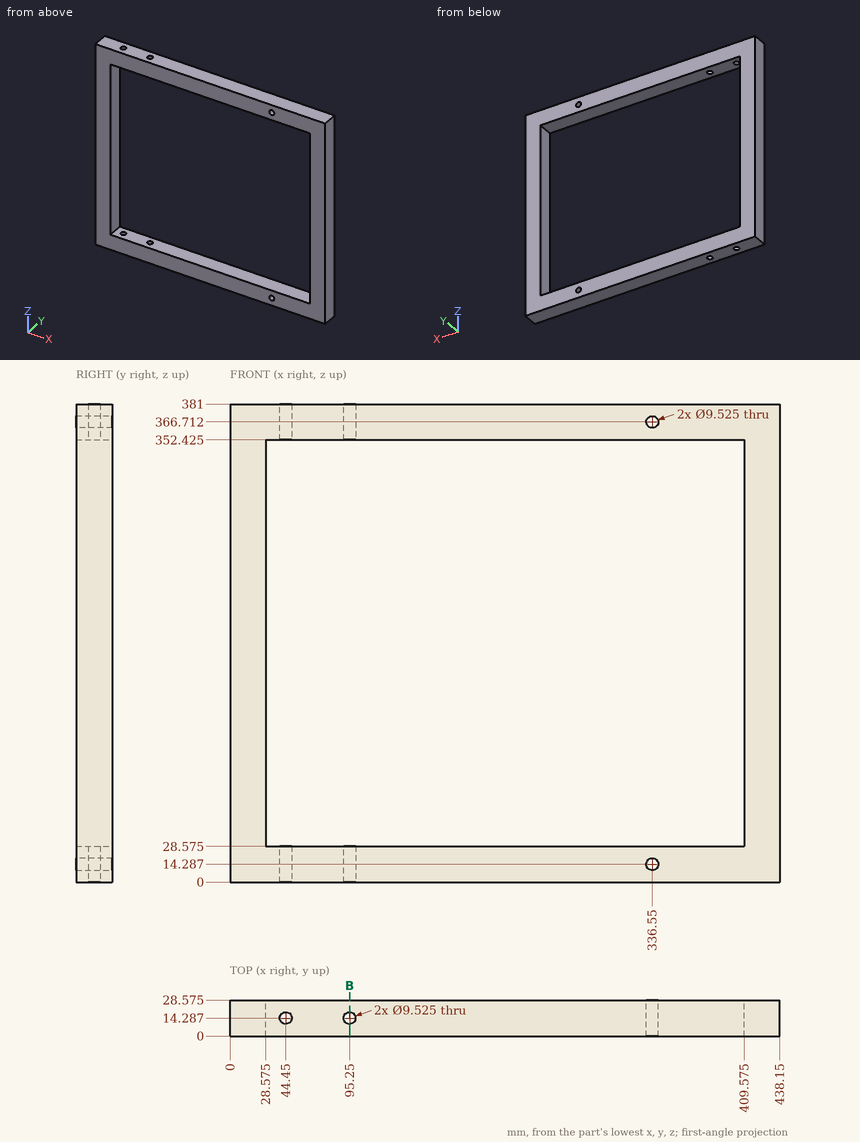
Geometry check sheet. Reference: drawing and pictorial views, mm from the part's lowest x, y, z. Round coordinates to 2 decimals unless told otherwise and drop trailing zeros. Use a Markdown table: item, result. Add a question column.
1. Thickness scan on probe 1 along Z at (x, y) = (291.5, 12.75) (1 decimal); probe 2 along Z at (x, y) = (333.5, 23.5) (1 decimal). Record the ranges inside material, lowest first. Write a range as [from, to].
2. Section check B-B, the plane x = 95.25. Give the number of separate pieces and of enclosed holes in the cut face, plus the area to 3 significant figures.
3. Gauge pin test, flat end, axial feed: pin 1 (1 mm diameter, centred on x = 93.5, y = 25, fed in from -Z). Record the tip position at first contact, or that the pin passes through.
Checks:
| question | item | result |
|---|---|---|
| 1 | probe 1 | z = [0, 28.6], [352.4, 381] |
| 1 | probe 2 | z = [0, 10.6], [17.9, 28.6], [352.4, 363.1], [370.4, 381] |
| 2 | separate pieces | 4 |
| 2 | enclosed holes | 0 |
| 2 | area | 1,090 mm^2 |
| 3 | pin 1 | stops at z = 0 |
